Check sheet for the modelled part. Datum: model origin and axes. Units: mm. A direction names the side the tool comes from. Round coordinates to 2 decimals unless told otherwise and drop trailing zeros. Order: outer loops, then holes, each group sorted by start corner. A loop starts at its lowest first (then second) coordinate and runs counter-clockwise, first axis right, second up. Notation, with made-up numbers: (-31, 73) -> (-9, 73) arc R25 cw to (-9, 98) -> close; hole circle Ø1 at (-6.5, 59.25). An arc over 180 degrees is marked (long way). Answer as CSV lines item,"result". Start each with the question number.
from build123d import *

# Parameters (mm, degrees)
F0_R     = 300
F0_W     = 20
F0_H     = 160
F0_R_2   = 30
F1_DEPTH = 20
F2_DEPTH = 700
F3_R     = 515
F4_DEPTH = 25


with BuildPart() as f1:
    # F0 (on Top) → F1 (new body)
    with BuildSketch(Plane.XY):
        Circle(F0_R)
        with Locations((0, -165)):
            Rectangle(F0_W, F0_H, mode=Mode.SUBTRACT)
        with Locations((-215, 0)):
            Circle(F0_R_2, mode=Mode.SUBTRACT)
        with Locations((215, 0)):
            Circle(F0_R_2, mode=Mode.SUBTRACT)
        with Locations((0, 165)):
            Rectangle(F0_W, F0_H, mode=Mode.SUBTRACT)
        with Locations((0, -165)):
            Rectangle(F0_W, F0_H)
        with Locations((0, 165)):
            Rectangle(F0_W, F0_H)
        with Locations((215, 0)):
            Circle(F0_R_2)
        with Locations((-215, 0)):
            Circle(F0_R_2)
    extrude(amount=-F1_DEPTH)

    # F0 (on Top) → F2 (join)
    with BuildSketch(Plane.XY):
        with Locations((215, 0)):
            Circle(F0_R_2)
        with Locations((-215, 0)):
            Circle(F0_R_2)
        with Locations((0, -165)):
            Rectangle(F0_W, F0_H)
        with Locations((0, 165)):
            Rectangle(F0_W, F0_H)
    extrude(amount=F2_DEPTH)

    # F3 (on face) → F4 (join)
    with BuildSketch(Plane.XY.offset(700)):
        Circle(F3_R)
    extrude(amount=F4_DEPTH)


solid = f1.part
1) Section check A-A on z = 106. Record the cut outline in (x, y), then the cut area to 3 significant figures.
2) Section check C-C on x = 215. Record the cut outline in (y, z), then the cut area to 3 significant figures.
3) Material ranges on line 1 along Z through (x, y) = (-37, 158.5); line 2 along X through (y, z) = (-210, 602.5); line 3 along Z through (x, y) = (343, -375), recorded low to high.
4) Depth check by flat-ended pin: pin 1 Ø6 at (x, y) = (269.5, -197.5) entering from -Z; pin 2 Ø22 at (x, z) = (-4, 445.5) entering from -Y; pin 3 Ø3 at (y, z) = (-1.5, 292) entering from -X. Enter the tip coordinate at first touch or a pass-through.
5) Section check B-B on y = 0. Record the cut outline in (x, z), then the cut area to 3 significant figures.
6) Section check D-D on y = -217.5. Record the cut outline in (x, z).
7) Mould release check, pull along Z, two halves, no side actions. Record for faces 1 (the face through (10, 164, 345)), 2 (the face through (-7, 7, 725)), 3 (the face through (-4, 4, -20)), 4 (the face through (-39.054, 297.447, -9.86)): released by +Z, released by -Z, zero draft, split by the parting line, or undercut.
8) Access from +Z, -Z, +X, -X, +Y, -Y to the whole of each face (thin tool, end or side, straight path). Record for faces 5 (the face through (-7, 7, 700)), 6 (the face through (10, -166, 345)), 7 (the face through (-10, 164, 345)).
Solutions:
1,outline,"circle Ø60 at (-215, 0); (-10, -245) -> (10, -245) -> (10, -85) -> (-10, -85) -> close; (-10, 85) -> (10, 85) -> (10, 245) -> (-10, 245) -> close; circle Ø60 at (215, 0)"
1,area,"12,100 mm^2"
2,outline,"(-467.97, 700) -> (-30, 700) -> (-30, 0) -> (-209.22, 0) -> (-209.22, -20) -> (209.22, -20) -> (209.22, 0) -> (30, 0) -> (30, 700) -> (467.97, 700) -> (467.97, 725) -> (-467.97, 725) -> close"
2,area,"73,800 mm^2"
3,line 1,"z = -20 to 0, 700 to 725"
3,line 2,"x = -10 to 10"
3,line 3,"z = 700 to 725"
4,pin 1,"stops at z = 700"
4,pin 2,"stops at y = -245"
4,pin 3,"stops at x = -245"
5,outline,"(-515, 700) -> (-245, 700) -> (-245, 0) -> (-300, 0) -> (-300, -20) -> (300, -20) -> (300, 0) -> (245, 0) -> (245, 700) -> (515, 700) -> (515, 725) -> (-515, 725) -> close; hole (-185, 0) -> (185, 0) -> (185, 700) -> (-185, 700) -> close"
5,area,"122,000 mm^2"
6,outline,"(-466.82, 700) -> (-10, 700) -> (-10, 0) -> (-206.62, 0) -> (-206.62, -20) -> (206.62, -20) -> (206.62, 0) -> (10, 0) -> (10, 700) -> (466.82, 700) -> (466.82, 725) -> (-466.82, 725) -> close"
7,face 1,"undercut"
7,face 2,"released by +Z"
7,face 3,"released by -Z"
7,face 4,"zero draft"
8,face 5,"none"
8,face 6,"+X, +Y, -Y"
8,face 7,"-X, +Y, -Y"
